Part model, mm, in its own coordinate system. A direction names the side the tool comes from. Coordinates: 2 decimals unless noted, no trailing zeros. Loops run counter-clockwise (first coordinate to the right, second up) from the corner with the lowest first, then second, coordinate; pieces in that order, holes last. Notation, with made-up numbers: (-35.75, -6) - (-18.75, -6) arc R11 ccw to (-18.75, 10) - close; hole circle Ø8 at (20, 32). An arc over 180 degrees is marked (long way). Use a Markdown table: item, result. Add a question column.
1. 3-axis set-ups, long thin cutter, end or side, ignore diameter. For faces 1 (the flat face through (-137.716, -9, -135)), 2 (the flat face through (14, -9, -331.715)), 3 (the flat face through (116.284, -9, -341)), 4 (the flat face through (-31.25, -9.39, -129.83)): which of +Z, -Z, +X, -X, +Y, -Y reach the whole face in a straight line?
2. Wall check: probe 1 along X at (y, z) = (-14.25, -290); probe 2 along X at (y, z) = (-1.5, 70); probe 3 along X at (y, z) = (-15.25, 130.5). Give the ranges that are in metal, low to high. Write a range as [from, to].
3. Band-saw the part on A-A, the plane x = -97. Give the cut face in (y, z).
4. Band-saw the part on B-B, the plane y = -10. Give the cut face in (x, z) (3 decimals).
5. Band-saw the part on D-D, the plane z = 141. Give the cut face in (x, y), plus the area to 3 significant figures.
6. Pull direction X, two halves, no side cores. Call faces 5 (the flat face through (38.517, -9.392, 74.154)), 6 (the flat face through (84, -9, -350.765)), 7 (the flat face through (-86.916, -9, -341)): pulls with the +X half, pulls with the -X half, needs draft (parallel to the pull), parting line crosses it, or undercut.
7. Drop flat-ended pins along their axis: pin 1 (8 mm diameter, centred on x = -90, y = -9, fed in from -Z); pin 2 (9.5 mm diameter, centred on y = -9, z = -345.5, fed in from +X); pin 3 (8 mm diameter, centred on x = 4.5, y = -12, fed in from -Z); pin 4 (9.5 mm diameter, centred on y = -6, z = -339, fed in from -X). Give the stop position or say it passes through.
8. Band-saw the part on C-C, the plane x = -34. Give the cut face in (y, z), plus the area to 3 significant figures.
from build123d import *

# Parameters (mm, degrees)
F1_DEPTH = 19.05


with BuildPart() as f1:
    # F0 (on Front) → F1 (new body)
    with BuildSketch(Plane.XZ):
        with BuildLine():
            Line((-137.715965, -183.12481), (-137.715965, -331.7148))
            Line((-137.715965, -331.7148), (-86.915965, -331.7148))
            Line((-86.915965, -331.7148), (-86.915965, -350.7648))
            Line((-86.915965, -350.7648), (-23.415965, -350.7648))
            Line((-23.415965, -350.7648), (-23.415965, -331.7148))
            Line((-23.415965, -331.7148), (52.784035, -331.7148))
            Line((52.784035, -331.7148), (52.784035, -350.7648))
            Line((52.784035, -350.7648), (116.284035, -350.7648))
            Line((116.284035, -350.7648), (116.284035, -331.7148))
            Line((116.284035, -331.7148), (167.084035, -331.7148))
            Line((167.084035, -331.7148), (167.084035, 245.768648))
            ThreePointArc((167.084035, 245.768648), (59.016129, 220.056395), (-25.892278, 148.4299))
            ThreePointArc((-25.892278, 148.4299), (-67.164643, 109.001513), (-116.097022, 79.613962))
            ThreePointArc((-116.097022, 79.613962), (-129.108758, 69.921843), (-137.715965, 56.168355))
            Line((-137.715965, 56.168355), (-137.715965, -183.12481))
        make_face()
        Polygon((-85.55314, -298.979528), (-103.454284, -292.464044), (-77.392349, -220.859466), (-59.656096, -227.827985), align=None, mode=Mode.SUBTRACT)
        Polygon((-22.508237, -133.262681), (-40.238813, -126.296393), (-12.373661, -55.374088), (5.356915, -62.340376), align=None, mode=Mode.SUBTRACT)
        Polygon((42.510451, 32.222697), (24.779875, 39.188985), (52.645027, 110.111289), (70.375603, 103.145001), align=None, mode=Mode.SUBTRACT)
    extrude(amount=F1_DEPTH)


solid = f1.part
Geometry check:
| question | item | result |
|---|---|---|
| 1 | face 1 | +Z, -Z, -X, +Y, -Y |
| 1 | face 2 | -Z, +Y, -Y |
| 1 | face 3 | -Z, +X, +Y, -Y |
| 1 | face 4 | +Y, -Y |
| 2 | probe 1 | x = [-137.72, -102.56], [-82.28, 167.08] |
| 2 | probe 2 | x = [-129.04, 36.89], [57.35, 167.08] |
| 2 | probe 3 | x = [-42.42, 167.08] |
| 3 | outline | (-19.05, -331.71) - (0, -331.71) - (0, -294.81) - (-19.05, -294.81) - close; (-19.05, -274.73) - (0, -274.73) - (0, 89.35) - (-19.05, 89.35) - close |
| 4 | outline | (-137.716, -331.715) - (-86.916, -331.715) - (-86.916, -350.765) - (-23.416, -350.765) - (-23.416, -331.715) - (52.784, -331.715) - (52.784, -350.765) - (116.284, -350.765) - (116.284, -331.715) - (167.084, -331.715) - (167.084, 245.769) arc R239.959 ccw to (-25.892, 148.43) arc R257.976 cw to (-116.097, 79.614) arc R43.938 ccw to (-137.716, 56.168) - close; hole (-103.454, -292.464) - (-85.553, -298.98) - (-59.656, -227.828) - (-77.392, -220.859) - close; hole (-40.239, -126.296) - (-22.508, -133.263) - (5.357, -62.34) - (-12.374, -55.374) - close; hole (24.78, 39.189) - (42.51, 32.223) - (70.376, 103.145) - (52.645, 110.111) - close |
| 5 | outline | (-32.36, -19.05) - (167.08, -19.05) - (167.08, 0) - (-32.36, 0) - close |
| 5 | area | 3,800 mm^2 |
| 6 | face 5 | undercut |
| 6 | face 6 | needs draft |
| 6 | face 7 | pulls with the -X half |
| 7 | pin 1 | stops at z = -350.76 |
| 7 | pin 2 | stops at x = 116.28 |
| 7 | pin 3 | stops at z = -331.71 |
| 7 | pin 4 | stops at x = -86.92 |
| 8 | outline | (-19.05, -350.76) - (0, -350.76) - (0, -128.75) - (-19.05, -128.75) - close; (-19.05, -110.42) - (0, -110.42) - (0, 139.21) - (-19.05, 139.21) - close |
| 8 | area | 8,980 mm^2 |
